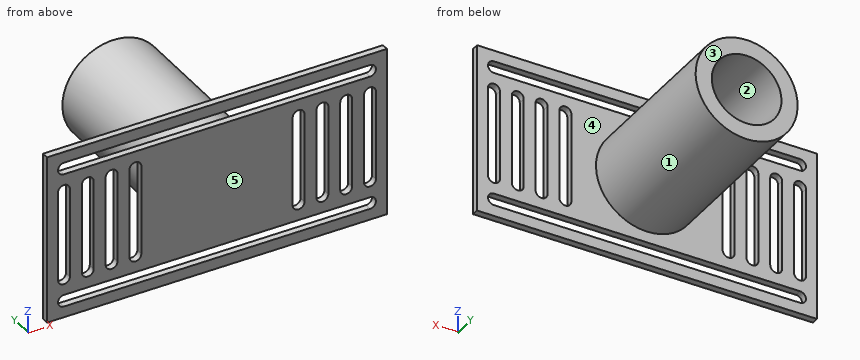
from build123d import *

# Parameters (mm, degrees)
SKETCH_1_W          = 100
SKETCH_1_H          = 50
EXTRUDE_1_DEPTH     = 2
SKETCH_2_R          = 15
SKETCH_2_R_2        = 10.25
EXTRUDE_2_DEPTH     = 50
CUT_EXTRUDE_1_DEPTH = 30


with BuildPart() as part:
    # 草图1 → 凸台-拉伸1 (new body)
    with BuildSketch(Plane(origin=(0, 0, 0), x_dir=(1, 0, 0), z_dir=(0, 1, 0))):
        with Locations((51.31061599, 25)):
            Rectangle(SKETCH_1_W, SKETCH_1_H)
    extrude(amount=EXTRUDE_1_DEPTH)

    # 草图2 → 凸台-拉伸2 (add)
    with BuildSketch(Plane(origin=(0, 2, 0), x_dir=(1, 0, 0), z_dir=(0, 1, 0))):
        with Locations(Location((51.31061599, 25, 0), (0, 0, 90))):
            Circle(SKETCH_2_R)
        with Locations(Location((51.31061599, 25, 0), (0, 0, 270))):
            Circle(SKETCH_2_R_2, mode=Mode.SUBTRACT)
    extrude(amount=EXTRUDE_2_DEPTH)

    # 草图3 → 切除-拉伸1 (cut)
    with BuildSketch(Plane.XZ):
        with BuildLine():
            Line((6.31061599, -3.25), (96.31061599, -3.25))
            ThreePointArc((96.31061599, -3.25), (98.06061599, -5), (96.31061599, -6.75))
            Line((96.31061599, -6.75), (6.31061599, -6.75))
            ThreePointArc((6.31061599, -6.75), (4.56061599, -5), (6.31061599, -3.25))
        make_face()
        with BuildLine():
            Line((6.31061599, -46.75), (96.31061599, -46.75))
            ThreePointArc((96.31061599, -46.75), (98.06061599, -45), (96.31061599, -43.25))
            Line((96.31061599, -43.25), (6.31061599, -43.25))
            ThreePointArc((6.31061599, -43.25), (4.56061599, -45), (6.31061599, -46.75))
        make_face()
        with BuildLine():
            Line((8.06061599, -11.75), (8.06061599, -38.25))
            ThreePointArc((8.06061599, -38.25), (6.31061599, -40), (4.56061599, -38.25))
            Line((4.56061599, -38.25), (4.56061599, -11.75))
            ThreePointArc((4.56061599, -11.75), (6.31061599, -10), (8.06061599, -11.75))
        make_face()
        with BuildLine():
            Line((94.56061599, -11.75), (94.56061599, -38.25))
            ThreePointArc((94.56061599, -38.25), (96.31061599, -40), (98.06061599, -38.25))
            Line((98.06061599, -38.25), (98.06061599, -11.75))
            ThreePointArc((98.06061599, -11.75), (96.31061599, -10), (94.56061599, -11.75))
        make_face()
        with BuildLine():
            Line((15.06061599, -11.75), (15.06061599, -38.25))
            ThreePointArc((15.06061599, -38.25), (13.31061599, -40), (11.56061599, -38.25))
            Line((11.56061599, -38.25), (11.56061599, -11.75))
            ThreePointArc((11.56061599, -11.75), (13.31061599, -10), (15.06061599, -11.75))
        make_face()
        with BuildLine():
            Line((22.06061599, -11.75), (22.06061599, -38.25))
            ThreePointArc((22.06061599, -38.25), (20.31061599, -40), (18.56061599, -38.25))
            Line((18.56061599, -38.25), (18.56061599, -11.75))
            ThreePointArc((18.56061599, -11.75), (20.31061599, -10), (22.06061599, -11.75))
        make_face()
        with BuildLine():
            Line((29.06061599, -11.75), (29.06061599, -38.25))
            ThreePointArc((29.06061599, -38.25), (27.31061599, -40), (25.56061599, -38.25))
            Line((25.56061599, -38.25), (25.56061599, -11.75))
            ThreePointArc((25.56061599, -11.75), (27.31061599, -10), (29.06061599, -11.75))
        make_face()
        with BuildLine():
            Line((87.56061599, -11.75), (87.56061599, -38.25))
            ThreePointArc((87.56061599, -38.25), (89.31061599, -40), (91.06061599, -38.25))
            Line((91.06061599, -38.25), (91.06061599, -11.75))
            ThreePointArc((91.06061599, -11.75), (89.31061599, -10), (87.56061599, -11.75))
        make_face()
        with BuildLine():
            Line((80.56061599, -11.75), (80.56061599, -38.25))
            ThreePointArc((80.56061599, -38.25), (82.31061599, -40), (84.06061599, -38.25))
            Line((84.06061599, -38.25), (84.06061599, -11.75))
            ThreePointArc((84.06061599, -11.75), (82.31061599, -10), (80.56061599, -11.75))
        make_face()
        with BuildLine():
            Line((73.56061599, -11.75), (73.56061599, -38.25))
            ThreePointArc((73.56061599, -38.25), (75.31061599, -40), (77.06061599, -38.25))
            Line((77.06061599, -38.25), (77.06061599, -11.75))
            ThreePointArc((77.06061599, -11.75), (75.31061599, -10), (73.56061599, -11.75))
        make_face()
    extrude(amount=-CUT_EXTRUDE_1_DEPTH, mode=Mode.SUBTRACT)


solid = part.part
Here's how the part is built. I have some questions about the finished solid (model axes, mm). Face numbers are marked on the shaded views. A direction names the side the tool comes from. Round coordinates to 2 decimals unless told otherwise and drop trailing zeros. Write each loop counter-clockwise with the first axis right and the second up, starting at its lowest first coordinate (ties: lowest second). Pieces come first, ordered by that corner, then holes.
1. For the marked faces 4 and 5, which set-ups out of +Z, -Z, +X, -X, +Y, -Y let a thin tool reach every point of the face, with its end or its side?
2. Suppose I cut it at B-B (x = 23.5). List the corners of the cut face in (y, z) for me, and give its area (3 significant figures).
3. If we mould it in two halves opening along Z, with no side actions, what happens to the marked faces 1, 2 and 3? For each: released by +Z, released by -Z, zero draft, split by the parting line, or undercut.
4. Suppose I cut it at C-C (z = -37). State how many separate pieces and enclosed holes the cut face has, and give its area (3 significant figures).
5. Suppose I cut it at A-A (z = -45). List the corners of the cut face in (x, y) for me.
6. I need wall thicknesses on L1, parallel to X at y = 20, z = -25; L2, parallel to Z at x = 51.5, y = 18; L3, parallel to Y at x = 18.5, z = -31. Which ranges of each line are inside material? Lowest first, please.
7. Will these pins go through, and if not, where does the flat tip stop? pin 1 Ø1 at (x, z) = (66.5, -21) entering from +Y; pin 2 Ø5 at (x, y) = (43, 21.5) entering from -Z; pin 3 Ø6 at (x, y) = (36, 27) entering from -Z.
8. Suppose I cut it at D-D (y = 29). List the corners of the cut face in (x, z) for me.
Answer sheet:
1. face 4: +Y
1. face 5: +Z, -Z, +X, -X, -Y
2. outline: (0, -50) - (2, -50) - (2, -46.75) - (0, -46.75) - close; (0, -43.25) - (2, -43.25) - (2, -6.75) - (0, -6.75) - close; (0, -3.25) - (2, -3.25) - (2, 0) - (0, 0) - close
2. area: 86.0 mm2
3. face 1: split by the parting line
3. face 2: undercut
3. face 3: zero draft
4. separate pieces: 9
4. enclosed holes: 0
4. area: 1,040 mm2
5. outline: (1.31, 0) - (4.56, 0) - (4.56, 2) - (1.31, 2) - close; (98.06, 0) - (101.31, 0) - (101.31, 2) - (98.06, 2) - close
6. L1: x = 36.31 to 41.06, 61.56 to 66.31
6. L2: z = -40 to -35.25, -14.75 to -10
6. L3: y = 0 to 2
7. pin 1: stops at y = 2
7. pin 2: stops at z = -38.83
7. pin 3: stops at z = -33.57
8. outline: circle Ø30 at (51.31, -25); hole circle Ø20.5 at (51.31, -25)
